Work out the finished part from the listing and answer in its coordinate system (mm). Round coordinates to 2 decimals unless told otherwise and drop trailing zeros. Loops run counter-clockwise (first coordinate to the right, second up) from the corner with the lowest first, then second, coordinate; pieces in that order, holes last. Notation, with made-up numbers: (89, 19) - (127, 19) arc R14 cw to (127, 38) - close; hole circle Ø11 at (6.5, 80.25). An arc over 180 degrees is marked (long way). Answer as CSV lines item,"result". Start each with the question number.
Q1. Section B-B on y = 35 is taken. Write down the section's boundary in (x, z), then the cut area to 3 significant figures.
Q2. Section D-D on y = 5 is taken. Write down the section's boundary in (x, z), then the cut area to 3 significant figures.
Q3. This flat-tipped pin is pushed along its axis until it touches: pin 1 Ø2.5 at (x, y) = (20, 5) entering from +Z. Where does it stop, or does it pass through?
Q4. Section A-A on x = 0 is taken. Write down the section's boundary in (y, z), then the cut area to 3 significant figures.
Q5. Section C-C on x = -20 is taken. Write down the section's boundary in (y, z), then the cut area to 3 significant figures.
Q6. The mould has two halves that part along Y. Classify faces 1 (the face through (-1, 53, 2)), 2 (the face through (18.73, 4.03, 0.99)), 3 (the face through (-41.76, 3.58, 0.99)): +Y half, -Y half, draft (parallel to the pull), parting line (faces both ways), or undercut.
Q7. Straight lines are drawn through the part: L1, parallel to X at y = 100, z = 0.65; L2, parallel to Y at x = 20, z = 1.5; L3, parallel to Y at x = -42.5, z = 1.1. For each, find the intervals that lie inside material, in ascending order. Write a range as [from, to].
```python
from build123d import *

# Parameters (mm, degrees)
SKETCH_1_R      = 1.6
SKETCH_1_W      = 50
SKETCH_1_H      = 30
EXTRUDE_3_DEPTH = 2


with BuildPart() as part:
    # 草圖1 → 填料-伸長3 (new body)
    # profile 1 of 2: a face of its own
    with BuildSketch(Plane.XY):
        Polygon((-47.5, 105), (-47.5, 0), (-25, 0), (-25, 30), (25, 30), (25, 0), (47.5, 0), (47.5, 105), align=None)
        with Locations((-42.5, 5)):
            Circle(SKETCH_1_R, mode=Mode.SUBTRACT)
        with Locations((42.5, 5)):
            Circle(SKETCH_1_R, mode=Mode.SUBTRACT)
        with Locations((0, 35)):
            Circle(SKETCH_1_R, mode=Mode.SUBTRACT)
        with Locations((-42.5, 100)):
            Circle(SKETCH_1_R, mode=Mode.SUBTRACT)
        with Locations((42.5, 100)):
            Circle(SKETCH_1_R, mode=Mode.SUBTRACT)
    # profile 2 of 2: a face of its own
    with BuildSketch(Plane.XY):
        with Locations((0, 15)):
            Rectangle(SKETCH_1_W, SKETCH_1_H)
        with Locations((-20, 5)):
            Circle(SKETCH_1_R, mode=Mode.SUBTRACT)
        with Locations((-20, 25)):
            Circle(SKETCH_1_R, mode=Mode.SUBTRACT)
        with Locations((20, 5)):
            Circle(SKETCH_1_R, mode=Mode.SUBTRACT)
        with Locations((20, 25)):
            Circle(SKETCH_1_R, mode=Mode.SUBTRACT)
    extrude(amount=EXTRUDE_3_DEPTH)


solid = part.part
```
Findings:
1,outline,"(-47.5, 0) - (-1.6, 0) - (-1.6, 2) - (-47.5, 2) - close; (1.6, 0) - (47.5, 0) - (47.5, 2) - (1.6, 2) - close"
1,area,"184 mm^2"
2,outline,"(-47.5, 0) - (-44.1, 0) - (-44.1, 2) - (-47.5, 2) - close; (-40.9, 0) - (-21.6, 0) - (-21.6, 2) - (-40.9, 2) - close; (-18.4, 0) - (18.4, 0) - (18.4, 2) - (-18.4, 2) - close; (21.6, 0) - (40.9, 0) - (40.9, 2) - (21.6, 2) - close; (44.1, 0) - (47.5, 0) - (47.5, 2) - (44.1, 2) - close"
2,area,"164 mm^2"
3,pin 1,"passes through"
4,outline,"(0, 0) - (33.4, 0) - (33.4, 2) - (0, 2) - close; (36.6, 0) - (105, 0) - (105, 2) - (36.6, 2) - close"
4,area,"204 mm^2"
5,outline,"(0, 0) - (3.4, 0) - (3.4, 2) - (0, 2) - close; (6.6, 0) - (23.4, 0) - (23.4, 2) - (6.6, 2) - close; (26.6, 0) - (105, 0) - (105, 2) - (26.6, 2) - close"
5,area,"197 mm^2"
6,face 1,"draft"
6,face 2,"undercut"
6,face 3,"undercut"
7,L1,"x = [-47.5, -44.1], [-40.9, 40.9], [44.1, 47.5]"
7,L2,"y = [0, 3.4], [6.6, 23.4], [26.6, 105]"
7,L3,"y = [0, 3.4], [6.6, 98.4], [101.6, 105]"
